The drawing under review shows one solid part. Ordinate dimensions are in mm from its lowest x, y, z. Coordinates: 2 decimals unless noted, no trailing zeros. Loops run counter-clockwise (first coordinate to the right, second up) from the corner with the lowest first, then second, coordinate; pieces in that order, holes last. Notation, with made-up numbers: (-22, 86) - (11, 86) arc R19 ccw to (11, 109) - close; hole circle Ø1 at (-25.75, 24.25). An arc over 180 degrees is marked (long way). Answer as a JSON object with one key per item and string values. Group by question number.
Item 1: To check wall thickness, follow line 1 (Z direction, x = 18, y = 8.75); line 2 (X direction, y = 6.75, z = 1.2); line 3 (X direction, y = 5.75, z = 3.7). State the ranges of each line that lie inside material, in increasing order.
Item 2: We need section A-A (y = 4.5). Give the boundary of the cut face in (x, z), then the cut area to 3 significant figures.
Item 3: Clearance check with flat-ended pins moving along their axes: pin 1 (2.5 mm diameter, centred on x = 13, y = 4, fed in from +Z); pin 2 (3.5 mm diameter, centred on x = 13.5, y = 8, fed in from +Z); pin 3 (1 mm diameter, centred on y = 3, z = 1, fed in from -X) (1 decimal); pin 4 (3 mm diameter, centred on y = 2.5, z = 2.5, fed in from -X) (1 decimal). State where each tip first meets the part, or that it passes through.
Item 4: We need section C-C (z = 1.8). Give the boundary of the cut face in (x, y) (1 decimal), then the cut area to 3 significant figures.
Item 5: We need section D-D (y = 7.5). Give the boundary of the cut face in (x, z).
Item 6: Mouldability with a two-part tool opening along X and no side actions: class the marked faces 1, 2 and 3 as released by +X, released by -X, zero draft, split by the parting line, or undercut.
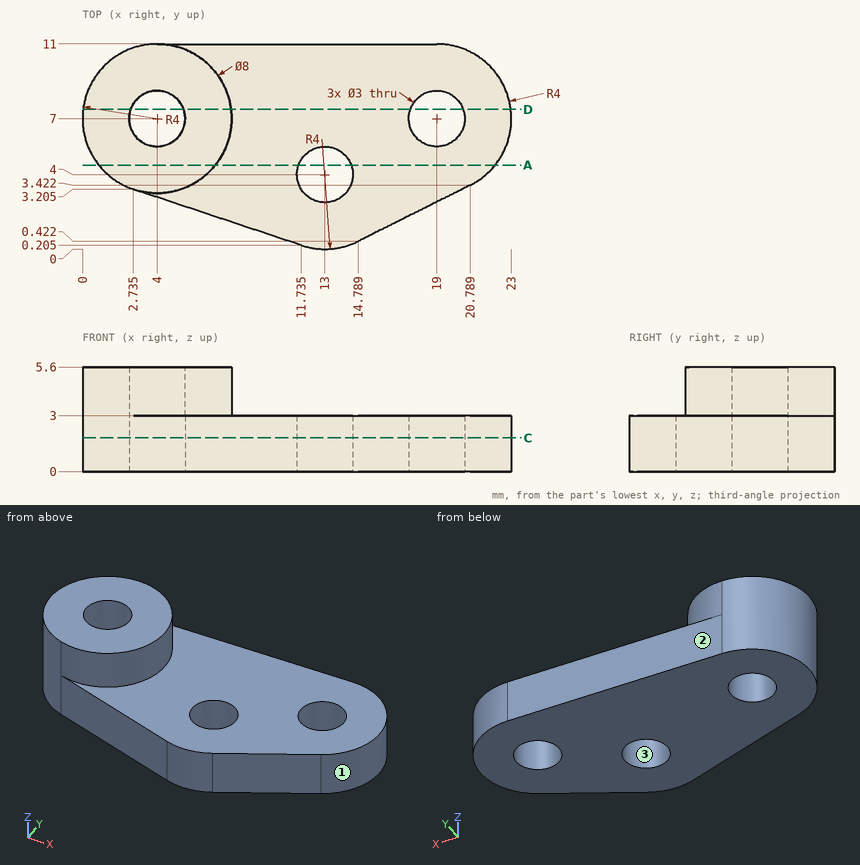
Check sheet entries:
{
 "1": {"line 1": "z = 0 to 3", "line 2": "x = 0.01 to 2.52, 5.48 to 17.52, 20.48 to 22.99", "line 3": "x = 0.2 to 3.17, 4.83 to 7.8"},
 "2": {"outline": "(0.88, 0) - (11.59, 0) - (11.59, 3) - (7.12, 3) - (7.12, 5.6) - (0.88, 5.6) - close; (14.41, 0) - (22.12, 0) - (22.12, 3) - (14.41, 3) - close", "area": "71.5 mm2"},
 "3": {"pin 1": "passes through", "pin 2": "stops at z = 3", "pin 3": "stops at x = 2.1", "pin 4": "stops at x = 1.4"},
 "4": {"outline": "(2.7, 3.2) - (11.7, 0.2) arc R4 ccw to (14.8, 0.4) - (20.8, 3.4) arc R4 ccw to (19, 11) - (4, 11) arc R4 ccw to start; hole circle Ø3 at (4, 7); hole circle Ø3 at (13, 4); hole circle Ø3 at (19, 7)", "area": "176 mm2"},
 "5": {"outline": "(0.03, 0) - (2.59, 0) - (2.59, 5.6) - (0.03, 5.6) - close; (5.41, 0) - (17.59, 0) - (17.59, 3) - (7.97, 3) - (7.97, 5.6) - (5.41, 5.6) - close; (20.41, 0) - (22.97, 0) - (22.97, 3) - (20.41, 3) - close"},
 "6": {"face 1": "released by +X", "face 2": "zero draft", "face 3": "undercut"}
}
